```python
from build123d import *

# Parameters (mm, degrees)
SKETCH1_W              = 184.15
SKETCH1_H              = 39.878
BOSS_EXTRUDE1_DEPTH    = 7.874
F_10_32_TAPPED_HOLE1_D = 4.0386
BOSS_EXTRUDE2_DEPTH    = 2.032


with BuildPart() as part:
    # Sketch1 → Boss-Extrude1 (new body)
    with BuildSketch(Plane(origin=(0, 0, 0), x_dir=(0, 0, -1), z_dir=(1, 0, 0))):
        Rectangle(SKETCH1_W, SKETCH1_H)
        with BuildLine():
            Line((-80.27524839, 6.6675), (80.27524839, 6.6675))
            ThreePointArc((80.27524839, 6.6675), (86.94274839, 0), (80.27524839, -6.6675))
            Line((80.27524839, -6.6675), (-80.27524839, -6.6675))
            ThreePointArc((-80.27524839, -6.6675), (-86.94274839, 0), (-80.27524839, 6.6675))
        make_face(mode=Mode.SUBTRACT)
    extrude(amount=BOSS_EXTRUDE1_DEPTH)

    # #10-32 Tapped Hole1 (through all)
    with Locations(Plane(origin=(7.874, 0, 0), x_dir=(0, 0, -1), z_dir=(1, 0, 0))):
        with Locations((-85.725, 13.589), (-85.725, -13.589), (0, -13.589), (85.725, -13.589), (85.725, 13.589), (0, 13.589)):
            Hole(F_10_32_TAPPED_HOLE1_D / 2)

    # Sketch5 → Boss-Extrude2 (add)
    with BuildSketch(Plane.ZY):
        with BuildLine():
            ThreePointArc((-80.27524839, 6.6675), (-73.60774839, 0), (-80.27524839, -6.6675))
            Line((-80.27524839, -6.6675), (-29.47524839, -6.6675))
            ThreePointArc((-29.47524839, -6.6675), (-36.14274839, -3e-09), (-29.475248395, 6.6675))
            Line((-29.475248395, 6.6675), (-80.27524839, 6.6675))
        make_face()
        with BuildLine():
            ThreePointArc((-22.80774839, 0), (-24.760613926, -4.714634464), (-29.47524839, -6.6675))
            Line((-29.47524839, -6.6675), (80.27524839, -6.6675))
            ThreePointArc((80.27524839, -6.6675), (86.94274839, 0), (80.27524839, 6.6675))
            Line((80.27524839, 6.6675), (-29.475248395, 6.6675))
            ThreePointArc((-29.475248395, 6.6675), (-24.760613928, 4.714634465), (-22.80774839, 0))
        make_face()
    extrude(amount=-BOSS_EXTRUDE2_DEPTH)


solid = part.part
```
Verification items for the finished model (mm, model axes). A direction names the side the tool comes from. Coordinates: 2 decimals unless noted, no trailing zeros. Loops run counter-clockwise (first coordinate to the right, second up) from the corner with the lowest first, then second, coordinate; pieces in that order, holes last. Notation, with made-up numbers: (-6, -19.5) -> (22, -19.5) arc R31 cw to (22, 16.5) -> close; hole circle Ø8 at (64, 52). An arc over 180 degrees is marked (long way). Answer in a Markdown table with one row per item. Add a question column.
1. Section check B-B, the plane y = -4. Enter the section's corners in (x, z) (3 decimals), then the cut area to 3 significant figures.
2. Section check C-C, the plane z = 69. Enter the section's corners in (x, y).
3. Section check A-A, the plane z = 0. Enter the section's corners in (x, y).
4. Section check D-D, the plane z = -27.5. Enter the section's corners in (x, y).
5. Material ranges on probe 1 along Z at (x, y) = (0.5, 0) (3 decimals); probe 2 along Y at (x, z) = (7, -43.5); probe 3 along Z at (x, y) = (1.75, 2) (3 decimals), recorded low to high. Write a range as [from, to].
6. Access from +Z, -Z, +X, -X, +Y, -Y to the whole of each face (thin tool, end or side, straight path). Record for faces 1 (the face through (4, -19.939, 1)), 2 (the face through (4.91, -0.15, 86.94)).
7. Draft check along Y on faces 3 (the face through (4, 0, 92.075)), 4 (the face through (4, 19.939, 1)), 5 (the face through (5, -6.668, -1)). Enter one of: +Y half, -Y half, draft (parallel to the pull), parting line (faces both ways), or undercut.
8. Depth check by flat-ended pin: P1, Ø6.5, axis at y = 1, z = 21, coming from the +X side. Enter the tip coordinate at first touch or a pass-through.
Derived:
| question | item | result |
|---|---|---|
| 1 | outline | (0, -92.075) -> (7.874, -92.075) -> (7.874, -85.61) -> (0, -85.61) -> close; (0, -74.941) -> (2.032, -74.941) -> (2.032, -34.81) -> (0, -34.81) -> close; (0, -24.141) -> (2.032, -24.141) -> (2.032, 85.61) -> (7.874, 85.61) -> (7.874, 92.075) -> (0, 92.075) -> close |
| 1 | area | 406 mm² |
| 2 | outline | (0, -19.94) -> (7.87, -19.94) -> (7.87, -6.67) -> (2.03, -6.67) -> (2.03, 6.67) -> (7.87, 6.67) -> (7.87, 19.94) -> (0, 19.94) -> close |
| 3 | outline | (0, -19.94) -> (7.87, -19.94) -> (7.87, -15.61) -> (0, -15.61) -> close; (0, -11.57) -> (7.87, -11.57) -> (7.87, -6.67) -> (2.03, -6.67) -> (2.03, 6.67) -> (7.87, 6.67) -> (7.87, 11.57) -> (0, 11.57) -> close; (0, 15.61) -> (7.87, 15.61) -> (7.87, 19.94) -> (0, 19.94) -> close |
| 4 | outline | (0, -19.94) -> (7.87, -19.94) -> (7.87, -6.67) -> (2.03, -6.67) -> (2.03, -6.37) -> (0, -6.37) -> close; (0, 6.37) -> (2.03, 6.37) -> (2.03, 6.67) -> (7.87, 6.67) -> (7.87, 19.94) -> (0, 19.94) -> close |
| 5 | probe 1 | z = [-92.075, -86.943], [-73.608, -36.143], [-22.808, 92.075] |
| 5 | probe 2 | y = [-19.94, -6.67], [6.67, 19.94] |
| 5 | probe 3 | z = [-92.075, -86.636], [-73.915, -35.836], [-23.115, 92.075] |
| 6 | face 1 | +Z, -Z, +X, -X, -Y |
| 6 | face 2 | +X |
| 7 | face 3 | draft |
| 7 | face 4 | +Y half |
| 7 | face 5 | undercut |
| 8 | P1 | stops at x = 2.03 |
